```python
from build123d import *

# Parameters (mm, degrees)
F1_DEPTH = 300
F2_T     = -4
F4_DEPTH = 25
F5_W     = 300
F5_H     = 220
F6_DEPTH = 25


with BuildPart() as f1:
    # F0 (on Top) → F1 (new body)
    with BuildSketch(Plane.XY):
        with BuildLine():
            Line((205.635, 242.809), (-205.635, 242.809))
            ThreePointArc((-205.635, 242.809), (-229.3674, 227.138989), (-238.558, 200.226))
            Line((-238.558, 200.226), (-238.558, -200.226))
            ThreePointArc((-238.558, -200.226), (-229.3674, -227.138989), (-205.635, -242.809))
            Line((-205.635, -242.809), (205.635, -242.809))
            ThreePointArc((205.635, -242.809), (229.367438, -227.139018), (238.558, -200.226))
            Line((238.558, -200.226), (238.558, 200.226))
            ThreePointArc((238.558, 200.226), (229.367438, 227.139018), (205.635, 242.809))
        make_face()
    extrude(amount=F1_DEPTH)

    # F2
    f2_openings = [f1.faces().sort_by_distance(p)[0] for p in [
        (4e-06, 0, 0),
    ]]
    offset(amount=F2_T, openings=f2_openings)

    # F3 (on face) → F4 (cut)
    with BuildSketch(Plane(origin=(0, 0, 296), x_dir=(1, 0, 0), z_dir=(0, 0, -1))):
        with BuildLine():
            ThreePointArc((-205.110852, 238.809), (-226.355128, 224.494202), (-234.558, 200.226))
            Line((-234.558, 200.226), (-234.558, -200.226))
            ThreePointArc((-234.558, -200.226), (-226.355128, -224.494202), (-205.110852, -238.809))
            Line((-205.110852, -238.809), (205.110858, -238.809))
            ThreePointArc((205.110858, -238.809), (226.35513, -224.494207), (234.558, -200.226013))
            Line((234.558, -200.226013), (234.558, 200.226))
            ThreePointArc((234.558, 200.226), (226.35513, 224.4942), (205.110858, 238.809))
            Line((205.110858, 238.809), (-205.110852, 238.809))
        make_face()
    extrude(amount=-F4_DEPTH, mode=Mode.SUBTRACT)

    # F5 (on face) → F6 (cut)
    with BuildSketch(Plane(origin=(-238.558, 0, 0), x_dir=(0, -1, 0), z_dir=(-1, 0, 0))):
        with Locations((25.226, 150)):
            Rectangle(F5_W, F5_H)
    extrude(amount=-F6_DEPTH, mode=Mode.SUBTRACT)


solid = f1.part
```
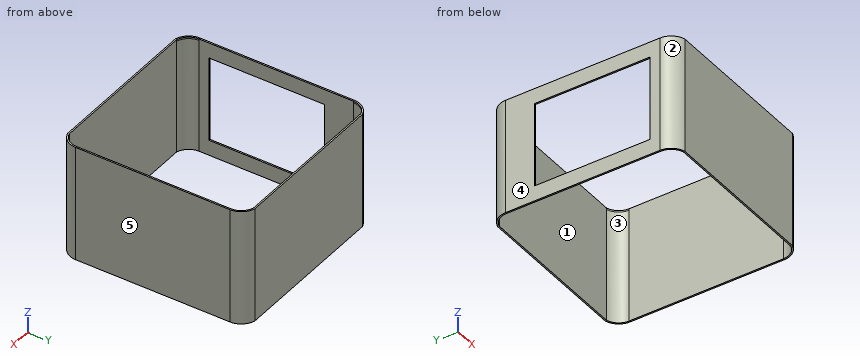
Build history of the part. All positions in model axes, mm. Face numbers are marked on the shaded views. A direction names the side the tool comes from. Give positions to 0.01 mm unless a question says otherwise; leave off trailing zeros. Loops run counter-clockwise (first coordinate to the right, second up) from the corner with the lowest first, then second, coordinate; pieces in that order, holes last. Notation, with made-up numbers: (81.5, -33) - (133.5, -33) arc R25 ccw to (133.5, -2) - close; hole circle Ø8 at (36, 28). An arc over 180 degrees is marked (long way). Use a Markdown table: item, result.
(1) Wall check: line 1 along X through (y, z) = (-179, 104.5); line 2 along Y through (x, z) = (-181.5, 169.5); line 3 along X through (y, z) = (74, 129). Give the ranges that are in metal, low to high.
Taken from the geometry:
| item | result |
|---|---|
| line 1 | -238.56 to -234.56, 234.56 to 238.56 |
| line 2 | -242.81 to -238.81, 238.81 to 242.81 |
| line 3 | 234.56 to 238.56 |
(2) Band-saw the part on C-C (z = 140). Give the cut face in (x, y) (3 decimals).
Taken from the geometry:
| item | result |
|---|---|
| outline | (-238.558, -200.226) arc R44 ccw to (-205.635, -242.809) - (205.635, -242.809) arc R44 ccw to (238.558, -200.226) - (238.558, 200.226) arc R44 ccw to (205.635, 242.809) - (-205.635, 242.809) arc R44 ccw to (-238.558, 200.226) - (-238.558, 124.774) - (-234.558, 124.774) - (-234.558, 200.226) arc R40 cw to (-205.111, 238.809) - (205.111, 238.809) arc R40 cw to (234.558, 200.226) - (234.558, -200.226) arc R40 cw to (205.111, -238.809) - (-205.111, -238.809) arc R40 cw to (-234.558, -200.226) - (-234.558, -175.226) - (-238.558, -175.226) - close |
(3) Band-saw the part on D-D (z = 32). Give the cut face in (x, y) (3 decimals).
Taken from the geometry:
| item | result |
|---|---|
| outline | (-238.558, -200.226) arc R44 ccw to (-205.635, -242.809) - (205.635, -242.809) arc R44 ccw to (238.558, -200.226) - (238.558, 200.226) arc R44 ccw to (205.635, 242.809) - (-205.635, 242.809) arc R44 ccw to (-238.558, 200.226) - close; hole (-234.558, -200.226) arc R40 ccw to (-205.111, -238.809) - (205.111, -238.809) arc R40 ccw to (234.558, -200.226) - (234.558, 200.226) arc R40 ccw to (205.111, 238.809) - (-205.111, 238.809) arc R40 ccw to (-234.558, 200.226) - close |
(4) Pull direction X, two halves, no side cores. Call the marked faces 3, 4 and 5: +X half, -X half, draft (parallel to the pull), parting line (faces both ways), or undercut.
Taken from the geometry:
| item | result |
|---|---|
| face 3 | undercut |
| face 4 | -X half |
| face 5 | +X half |
(5) Drop flat-ended pins along their axis: pin 1 Ø1.2 at (x, z) = (-236, 121.5) entering from +Y; pin 2 Ø5 at (y, z) = (73.5, 222.5) entering from -X. Give the stop position or say it passes through.
Taken from the geometry:
| item | result |
|---|---|
| pin 1 | y = 216.59 |
| pin 2 | x = 234.56 |
(6) Band-saw the part on B-B (x = -79.5). Give the cut face in (y, z).
Taken from the geometry:
| item | result |
|---|---|
| outline | (-242.81, 0) - (-238.81, 0) - (-238.81, 300) - (-242.81, 300) - close; (238.81, 0) - (242.81, 0) - (242.81, 300) - (238.81, 300) - close |
(7) Which spindle directions (+Z, -Z, +X, -X, +Y, -Y) get a long thin tool onto all of the face, cutting with end or side? Do the marked faces 1 and 2. Say none if no direction does.
Taken from the geometry:
| item | result |
|---|---|
| face 1 | +Z, -Z |
| face 2 | +Z, -Z, -X, -Y |
(8) Band-saw the part on A-A (y = -39). Give the cut face in (x, z).
Taken from the geometry:
| item | result |
|---|---|
| outline | (-238.56, 0) - (-234.56, 0) - (-234.56, 40) - (-238.56, 40) - close; (-238.56, 260) - (-234.56, 260) - (-234.56, 300) - (-238.56, 300) - close; (234.56, 0) - (238.56, 0) - (238.56, 300) - (234.56, 300) - close |
